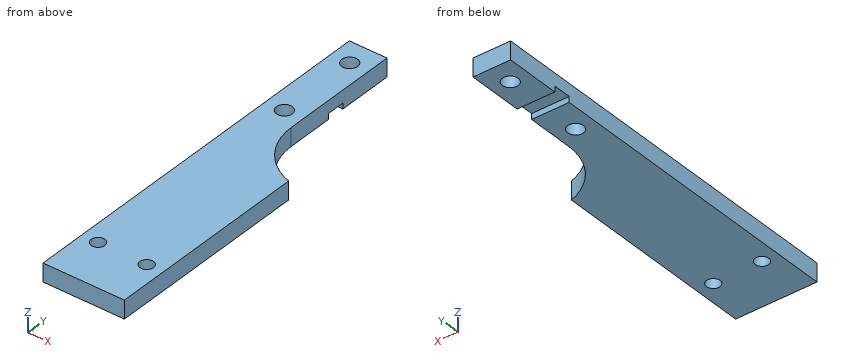
from build123d import *

# Parameters (mm, degrees)
PAD002_DEPTH    = 4
SKETCH008_R     = 1.75
SKETCH008_R_2   = 1.5
POCKET009_DEPTH = 5
SKETCH009_W     = 10.460062
SKETCH009_H     = 4
POCKET001_DEPTH = 1.25


with BuildPart() as part:
    # Sketch007 → Pad002 (new body)
    with BuildSketch(Plane.XY):
        with BuildLine():
            Line((-4.135, 20), (-4.135, -65))
            Line((-4.135, -65), (13.765, -65))
            Line((13.765, -65), (13.765, -19.428397))
            ThreePointArc((4.135, -6.621152), (6.848343, -14.605049), (13.765, -19.428397))
            Line((4.135, 20), (4.135, -6.621152))
            Line((4.135, 20), (-4.135, 20))
        make_face()
    extrude(amount=PAD002_DEPTH)

    # Sketch008 (on Face8 of Pad002) → Pocket009 (cut)
    with BuildSketch(Plane.XY.offset(4)):
        with Locations((0, 14.875)):
            Circle(SKETCH008_R)
        with Locations((0, -3.255)):
            Circle(SKETCH008_R)
        with Locations((-0.54, -54.255)):
            Circle(SKETCH008_R_2)
        with Locations((10.16, -54.255)):
            Circle(SKETCH008_R_2)
    extrude(amount=-POCKET009_DEPTH, mode=Mode.SUBTRACT)

    # Sketch009 (on Face4 of Pocket009) → Pocket001 (cut)
    with BuildSketch(Plane(origin=(0, 0, 0), x_dir=(1, 0, 0), z_dir=(0, 0, -1))):
        with Locations((-0.716524, -5.745)):
            Rectangle(SKETCH009_W, SKETCH009_H)
    extrude(amount=-POCKET001_DEPTH, mode=Mode.SUBTRACT)


solid = part.part
Source: CAD feature listing. Evaluate the final solid. Frame: model axes, mm. Round coordinates to 2 decimals unless told otherwise and drop trailing zeros. Order: outer loops, then holes, each group sorted by start corner. A loop starts at its lowest first (then second) coordinate and runs counter-clockwise, first axis right, second up. Notation, with made-up numbers: (16, 39) - (49, 39) arc R15 cw to (49, 44) - close; hole circle Ø8 at (47, -20.5). An arc over 180 degrees is marked (long way). Use a Markdown table: item, result. Add a question column.
1. Line query: probe 1 along Y at (x, z) = (1.5, 2.7); probe 2 along Y at (x, z) = (-2.75, 0.35) (3 decimals); probe 3 along Y at (x, z) = (0, 2.3) (3 decimals). Output: solid intervals per line, ascending.
2. Section query C-C (x = 6.75). Return the cut outline in (y, z), then the cut area to 3 significant figures.
3. First-contact query: pin 1 (1.2 mm diameter, centred on x = 1, y = 6.5, fed in from -Z); pin 2 (1.2 mm diameter, centred on y = 1, z = 2, fed in from +X) (3 decimals). Flat tips, straight axial feed; report the tip coordinate or a pass-through.
4. Section query B-B (x = 0). Return the cut outline in (y, z) (3 decimals).
5. Section query A-A (x = 10.25). Return the cut outline in (y, z), then the cut area to 3 significant figures.
Derived:
| question | item | result |
|---|---|---|
| 1 | probe 1 | -65 to -4.16, -2.35 to 13.97, 15.78 to 20 |
| 1 | probe 2 | -65 to 3.745, 7.745 to 20 |
| 1 | probe 3 | -65 to -55.654, -52.856 to -5.005, -1.505 to 13.125, 16.625 to 20 |
| 2 | outline | (-65, 0) - (-14.47, 0) - (-14.47, 4) - (-65, 4) - close |
| 2 | area | 202 mm2 |
| 3 | pin 1 | z = 1.25 |
| 3 | pin 2 | x = 4.135 |
| 4 | outline | (-65, 0) - (-55.654, 0) - (-55.654, 4) - (-65, 4) - close; (-52.856, 0) - (-5.005, 0) - (-5.005, 4) - (-52.856, 4) - close; (-1.505, 0) - (3.745, 0) - (3.745, 1.25) - (7.745, 1.25) - (7.745, 0) - (13.125, 0) - (13.125, 4) - (-1.505, 4) - close; (16.625, 0) - (20, 0) - (20, 4) - (16.625, 4) - close |
| 5 | outline | (-65, 0) - (-55.75, 0) - (-55.75, 4) - (-65, 4) - close; (-52.76, 0) - (-17.79, 0) - (-17.79, 4) - (-52.76, 4) - close |
| 5 | area | 177 mm2 |
